```python
from build123d import *

# Parameters (mm, degrees)
SKETCH1_W           = 20
SKETCH1_H           = 20
BOSS_EXTRUDE1_DEPTH = 1.5
FILLET1_R           = 1.5
SKETCH2_R           = 1.5
CUT_EXTRUDE1_DEPTH  = 1.5
SKETCH3_W           = 10
SKETCH3_H           = 7
BOSS_EXTRUDE2_DEPTH = 6
SKETCH4_W           = 13
SKETCH4_H           = 6.5
BOSS_EXTRUDE3_DEPTH = 6


with BuildPart() as part:
    # Sketch1 → Boss-Extrude1 (new body)
    with BuildSketch(Plane(origin=(0, 0, 0), x_dir=(1, 0, 0), z_dir=(0, 1, 0))):
        Rectangle(SKETCH1_W, SKETCH1_H)
    extrude(amount=BOSS_EXTRUDE1_DEPTH)

    # Fillet1
    fillet1_edges = [part.edges().sort_by_distance(p)[0] for p in [
        (-10, 0.75, -10),
        (10, 0.75, -10),
        (10, 0.75, 10),
        (-10, 0.75, 10),
    ]]
    fillet(fillet1_edges, radius=FILLET1_R)

    # Sketch2 → Cut-Extrude1 (cut)
    with BuildSketch(Plane(origin=(0, 1.5, 0), x_dir=(1, 0, 0), z_dir=(0, 1, 0))):
        with Locations(Location((7, 7, 0), (0, 0, 270))):
            Circle(SKETCH2_R)
        with Locations(Location((-7, 7, 0), (0, 0, 270))):
            Circle(SKETCH2_R)
    extrude(amount=-CUT_EXTRUDE1_DEPTH, mode=Mode.SUBTRACT)

    # Sketch3 → Boss-Extrude2 (add)
    with BuildSketch(Plane(origin=(0, 1.5, 0), x_dir=(1, 0, 0), z_dir=(0, 1, 0))):
        with Locations((0, 9.5)):
            Rectangle(SKETCH3_W, SKETCH3_H)
    extrude(amount=BOSS_EXTRUDE2_DEPTH)

    # Sketch4 → Boss-Extrude3 (add)
    with BuildSketch(Plane(origin=(0, 1.5, 0), x_dir=(1, 0, 0), z_dir=(0, 1, 0))):
        with Locations((-1.5, -8.75)):
            Rectangle(SKETCH4_W, SKETCH4_H)
    extrude(amount=BOSS_EXTRUDE3_DEPTH)


solid = part.part
```
Input: part model. Units: mm. Frame: model coordinates. A direction names the side the tool comes from. Coordinates: 2 decimals unless noted, no trailing zeros. Loops run counter-clockwise (first coordinate to the right, second up) from the corner with the lowest first, then second, coordinate; pieces in that order, holes last. Notation, with made-up numbers: (28, -7.5) - (87, -7.5) arc R31 ccw to (87, 28.5) - close; hole circle Ø3 at (1.5, 5.25). An arc over 180 degrees is marked (long way). Answer in a Markdown table with one row per item.
(1) Cut plane B-B on y = 5.75. Output: boundary loops of the cut face in (x, z).
Model answer:
| item | result |
|---|---|
| outline | (-8, 5.5) - (5, 5.5) - (5, 12) - (-8, 12) - close; (-5, -13) - (5, -13) - (5, -6) - (-5, -6) - close |
(2) Pin query (flat end, axial travel): P1, Ø1.5, axis at y = 2.5, z = -8.5, coming from the -X side; P2, Ø0.6, axis at x = -1, z = 11, coming from the -Y side; P3, Ø3, axis at x = 7, z = -1, coming from the +Y side. Return the tip coordinate at first contact, or that it passes through.
Model answer:
| item | result |
|---|---|
| P1 | stops at x = -5 |
| P2 | stops at y = 1.5 |
| P3 | stops at y = 1.5 |
(3) Cut plane A-A on z = -7. Output: boundary loops of the cut face in (x, y), plus the area to 3 significant figures.
Model answer:
| item | result |
|---|---|
| outline | (-10, 0) - (-8.5, 0) - (-8.5, 1.5) - (-10, 1.5) - close; (-5.5, 0) - (5.5, 0) - (5.5, 1.5) - (5, 1.5) - (5, 7.5) - (-5, 7.5) - (-5, 1.5) - (-5.5, 1.5) - close; (8.5, 0) - (10, 0) - (10, 1.5) - (8.5, 1.5) - close |
| area | 81.0 mm² |
(4) Cut plane C-C on x = -7. Output: boundary loops of the cut face in (y, z).
Model answer:
| item | result |
|---|---|
| outline | (0, -10) - (1.5, -10) - (1.5, -8.5) - (0, -8.5) - close; (0, -5.5) - (1.5, -5.5) - (1.5, 5.5) - (7.5, 5.5) - (7.5, 12) - (1.5, 12) - (1.5, 10) - (0, 10) - close |
(5) Material intervals for L1, parallel to X at y = 1.15, z = -7; L2, parallel to Z at x = -4, y = 1.75; L3, parallel to X at y = 6.75, z = 11, sorted ascending. Write a range as from..to.
Model answer:
| item | result |
|---|---|
| L1 | x = -10..-8.5, -5.5..5.5, 8.5..10 |
| L2 | z = -13..-6, 5.5..12 |
| L3 | x = -8..5 |
(6) Mould query, pull axis Z, two halves, no side actions, for faces 1 (the face through (-2, 1.5, 11)), 2 (the face through (0, 4, -13)), 3 (the face through (-2, 4, 5.5)), 4 (the face through (9.55, 0.76, 9.57)). Classes: pulls with the +Z half, pulls with the -Z half, needs draft (parallel to the pull), parting line crosses it, or undercut.
Model answer:
| item | result |
|---|---|
| face 1 | needs draft |
| face 2 | pulls with the -Z half |
| face 3 | undercut |
| face 4 | pulls with the +Z half |
(7) Set-up query: faces 5 (the face through (0, 4, -6)), 6 (the face through (5, 4, 9)), 7 (the face through (-5, 4, -9)). Return all of +Z, -Z, +X, -X, +Y, -Y with unobstructed straight access to the full face (end or side cutting, diameter ignored); none if empty.
Model answer:
| item | result |
|---|---|
| face 5 | +X, -X, +Y |
| face 6 | +Z, -Z, +X, +Y |
| face 7 | -Z, -X, +Y |
(8) Cut plane D-D on y = 0.75. Output: boundary loops of the cut face in (x, z), plus the area to 3 significant figures.
Model answer:
| item | result |
|---|---|
| outline | (-10, -8.5) arc R1.5 ccw to (-8.5, -10) - (8.5, -10) arc R1.5 ccw to (10, -8.5) - (10, 8.5) arc R1.5 ccw to (8.5, 10) - (-8.5, 10) arc R1.5 ccw to (-10, 8.5) - close; hole circle Ø3 at (-7, -7); hole circle Ø3 at (7, -7) |
| area | 384 mm² |
